Autodesk Inventor part; units mm, degrees
ref_plane "Work Plane1" through (0, -13.725, 0) normal (1, 0, 0) x (0, 0, 1)
ref_plane "YZ Plane" through (0, 0, 0) normal (1, 0, 0) x (0, 1, 0)
ref_plane "XZ Plane" through (0, 0, 0) normal (0, 1, 0) x (-1, 0, 0)
sketch "Szkic1" plane through (0, 0, 0) normal (0, 0, 1) x (1, 0, 0)
  arc A0 (9.4933, -21.8953) -> (-9.4933, -21.8953) centre (0, -13.725) ccw
  line L0 (0, 15.1128) -> (0, -73.1766)
  line L1 (-45.5, 0) -> (45.5, 0)
  line L2 (-4.9645, 1.7) -> (1.5024, 1.7) construction
  arc A1 (4.998, -26.8243) -> (-4.998, -26.8243) centre (0, -13) ccw
  line L3 (0, -1.2) -> (-5.3069, -1.2) construction
  line L4 (0, -13) -> (-6.8324, -26.0157) construction
  line L5 (-6.8324, -26.0157) -> (-20.0146, -19.0959) construction
  line L6 (-5.7169, -23.8907) -> (-15.9662, -18.5105) construction
  circle A2 centre (-5.7169, -23.8907) radius 1
  arc A3 (-3.946, -24.8203) -> (-6.8471, -22.2407) centre (-5.7169, -23.8907) ccw
  arc A4 (-9.4933, -21.8953) -> (-6.8471, -22.2407) centre (-7.9774, -20.5907) ccw
  line L7 (-3.946, -24.8203) -> (-4.998, -26.8243)
  circle A5 centre (5.7169, -23.8907) radius 1
  arc A6 (6.8471, -22.2407) -> (3.946, -24.8203) centre (5.7169, -23.8907) ccw
  arc A7 (6.8471, -22.2407) -> (9.4933, -21.8953) centre (7.9774, -20.5907) ccw
  line L8 (3.946, -24.8203) -> (4.998, -26.8243)
  point P0 (-13.0867, -20.022)
  point P1 (6.8324, -26.0157)
  dimension "d8" = 0.725
  dimension "d38" = 2.9
  dimension "d39" = 13
  dimension "d43" = 14.7
  dimension "d45" = 2.4
  dimension "d46" = 2
  dimension "d47" = 4.998
  dimension "d48" = 2
  dimension "d49" = 2
extrude "Bryła" add sketch "Szkic1" along normal blind 1.2
ref_plane "Work Plane1" through (0, -13.725, 0) normal (1, 0, 0) x (0, 0, 1)
equation "\"d8\" = 0.25 * SRB1"
equation "\"d38\" = SRB1"
equation "\"d39\" = 0.5 * WD"
equation "\"d43\" = 0.5 * ND"
equation "\"d45\" = 0.5 * SRB2"
equation "\"d46\" = SD5"
equation "\"d47\" = 0.17 * ND"
equation "\"d48\" = SD5"
equation "\"d49\" = SD5"
equation "\"d2\" = SD"
equation "\"WD\" = WDMIN"
equation "\"SD\" = 1.2"
equation "\"SRB1\" = 2.9"
equation "\"ND\" = 29.4"
equation "\"SRB2\" = 4.8"
equation "\"SD5\" = 2"
equation "\"WDMIN\" = 26"
equation "\"SD6\" = 30.1"
equation "\"NND\" = 28"
equation "\"WDMAX\" = NND"
properties part number "DIN 472 - 28 x 1,2" material "Stal, miękka"
Can you work these out from the model? Positions are in its coordinate system, mm. A direction names the side the tool comes from. Round coordinates to 2 decimals unless told otherwise and drop trailing zeros. Loops run counter-clockwise (first coordinate to the right, second up) from the corner with the lowest first, then second, coordinate; pieces in that order, holes last. Notation, with made-up numbers: (80.25, 50) -> (137.25, 50) arc R20 cw to (137.25, 76) -> close; hole circle Ø11 at (63.5, 41). An arc over 180 degrees is marked (long way). Answer in a Markdown table with one row per item.
Item 1: Suppose I cut it at D-D, the plane x = 0. List the corners of the cut face in (y, z) for me.
Answer block:
| item | result |
|---|---|
| outline | (-1.2, 0) -> (1.7, 0) -> (1.7, 1.2) -> (-1.2, 1.2) -> close |
Item 2: Suppose I cut it at A-A, the plane y = -21.5. List the corners of the cut face in (x, z) for me.
Answer block:
| item | result |
|---|---|
| outline | (-11.99, 0) -> (-9.82, 0) -> (-9.82, 1.2) -> (-11.99, 1.2) -> close; (9.82, 0) -> (11.99, 0) -> (11.99, 1.2) -> (9.82, 1.2) -> close |
Item 3: If I drill on probe 1 along Y at (x, z) = (6.25, 0.65); probe 2 along X at (y, z) = (-23.75, 1.1); probe 3 along X at (y, z) = (-12.75, 0.2), over which ranges is the centre line in solid material (lowest first)?
Answer block:
| item | result |
|---|---|
| probe 1 | -26.31 to -24.74, -23.04 to -21.96, -2.87 to 0.31 |
| probe 2 | -10.03 to -6.71, -4.73 to -3.72, 3.72 to 4.73, 6.71 to 10.03 |
| probe 3 | -14.7 to -12.49, 12.49 to 14.7 |
Item 4: Suppose I cut it at C-C, the plane z = 0.8. List the corners of the cut face in (x, y) for me (3 decimals), plus the area to 3 significant figures.
Answer block:
| item | result |
|---|---|
| outline | (-9.493, -21.895) arc R12.525 cw (long way) to (9.493, -21.895) arc R2 cw to (6.847, -22.241) arc R2 ccw to (3.946, -24.82) -> (4.998, -26.824) arc R14.7 ccw (long way) to (-4.998, -26.824) -> (-3.946, -24.82) arc R2 ccw to (-6.847, -22.241) arc R2 cw to start; hole circle Ø2 at (-5.717, -23.891); hole circle Ø2 at (5.717, -23.891) |
| area | 187 mm² |
Item 5: On a 3-axis mill with a long thin cutter (end or side, diameter ignored), from which of +Z, -Z, +X, -X, +Y, -Y can I reach the whole of each face in a straight line? I mean faces 1 (the cylindrical face through (8.26, -22.57, 0.59)), 2 (the flat face through (-1, -1, 1.2)), 3 (the flat face through (4.465, -25.808, 0.592)). Say none if no direction works.
Answer block:
| item | result |
|---|---|
| face 1 | +Z, -Z |
| face 2 | +Z, +X, -X, +Y, -Y |
| face 3 | +Z, -Z, -Y |
Item 6: Suppose I cut it at B-B, the plane x = -7.75. List the corners of the cut face in (y, z) for me, plus the area to 3 significant figures.
Answer block:
| item | result |
|---|---|
| outline | (-25.49, 0) -> (-22.58, 0) -> (-22.58, 1.2) -> (-25.49, 1.2) -> close; (-3.89, 0) -> (-0.51, 0) -> (-0.51, 1.2) -> (-3.89, 1.2) -> close |
| area | 7.55 mm² |
Item 7: Will this pin go through, and if not, where does the flat tip stop? P1, Ø6, axis at x = 3.5, y = -7, coming from the -Z side.
Answer block:
| item | result |
|---|---|
| P1 | through |
